Source: CAD feature listing. Evaluate the final solid. Frame: model axes, mm. Face numbers are marked on the shaded views. A direction names the side the tool comes from. Round coordinates to 2 decimals unless told otherwise and drop trailing zeros. Order: outer loops, then holes, each group sorted by start corner. A loop starts at its lowest first (then second) coordinate and runs counter-clockwise, first axis right, second up. Notation, with made-up numbers: M -40,-19 L 8,-19 A37 ccw 8,20 Z; hole C -2.75,52 d2. An arc over 180 degrees is marked long. Answer as CSV lines item,"result". Start each with the question number.
Item 1: Set-up query: the marked faces 1, 2, 3, 4 and 5. Return all of +Z, -Z, +X, -X, +Y, -Y with unobstructed straight access to the full face (end or side cutting, diameter ignored); none if empty.
Item 2: First-contact query: P1, Ø1, axis at x = -54, y = 23, coming from the +Z side; P2, Ø5.5, axis at x = -62.5, z = 3.5, coming from the -Y side; P3, Ø9, axis at x = -55, y = 24, coming from the -Z side; P4, Ø2, axis at y = 43.5, z = 7, coming from the +X side. Flat tips, straight axial feed; report the tip coordinate or a pass-through.
Item 3: Section query B-B on y = 5. Return the cut outline in (x, z), plus the area to 3 significant figures.
Item 4: Section query D-D on y = 24. Return the cut outline in (x, z).
Item 5: Section query C-C on x = -44. Return the cut outline in (y, z).
Item 6: Line query: line 1 (Z direction, x = -56.5, y = 35.5); line 2 (X direction, y = 54.5, z = 1.75); line 3 (Y direction, x = -68, z = 2). Output: solid intervals per line, ascending. Write a range as [from, to].
Item 7: Section query A-A on z = -0.75. Return the cut outline in (x, y), plus the area to 3 significant figures.
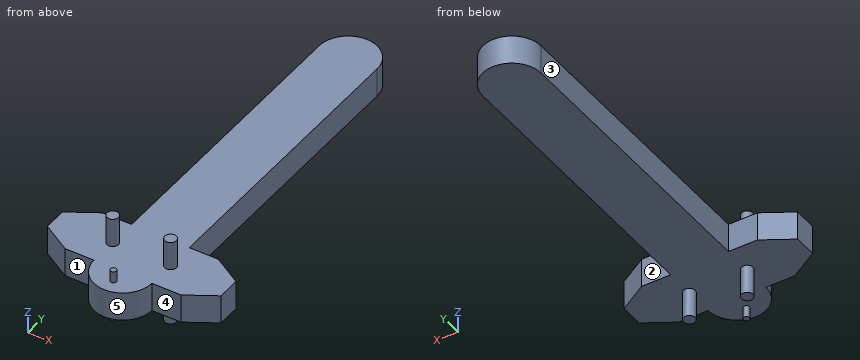
from build123d import *

# Parameters (mm, degrees)
F0_R     = 1
F0_R_2   = 0.5
F1_DEPTH = 5
F2_DEPTH = 7
F3_DEPTH = 2
F4_DEPTH = 10
F5_DEPTH = 5


with BuildPart() as f1:
    # F0 (on Top) → F1 (new body)
    with BuildSketch(Plane.XY):
        with BuildLine():
            Line((-60.480928, 60), (-60.480928, 10))
            Line((-60.480928, 10), (-50.480928, 10))
            Line((-50.480928, 10), (-50.480928, 60))
            ThreePointArc((-50.480928, 60), (-55.480928, 65), (-60.480928, 60))
        make_face()
        Polygon((-50.480928, 10), (-60.480928, 10), (-65.480928, 10), (-70.480928, 7), (-70.480928, 3), (-65.480928, 0), (-60.480928, 0), (-50.480928, 0), (-45.480928, 0), (-40.480928, 3), (-40.480928, 7), (-45.480928, 10), align=None)
        with Locations((-60.480928, 5)):
            Circle(F0_R, mode=Mode.SUBTRACT)
        with Locations((-50.480928, 5)):
            Circle(F0_R, mode=Mode.SUBTRACT)
        with BuildLine():
            Line((-50.480928, 0), (-60.480928, 0))
            ThreePointArc((-60.480928, 0), (-55.480928, -5), (-50.480928, 0))
        make_face()
        with Locations((-55.480928, -2.5)):
            Circle(F0_R_2, mode=Mode.SUBTRACT)
        with Locations((-55.480928, -2.5)):
            Circle(F0_R_2)
    extrude(amount=F1_DEPTH)

    # F0 (on Top) → F2 (join)
    with BuildSketch(Plane.XY):
        with Locations((-55.480928, -2.5)):
            Circle(F0_R_2)
    extrude(amount=F2_DEPTH)

    # F0 (on Top) → F3 (join)
    with BuildSketch(Plane.XY):
        with Locations((-55.480928, -2.5)):
            Circle(F0_R_2)
    extrude(amount=-F3_DEPTH)

    # F0 (on Top) → F4 (join)
    with BuildSketch(Plane.XY):
        with Locations((-60.480928, 5)):
            Circle(F0_R)
        with Locations((-50.480928, 5)):
            Circle(F0_R)
    extrude(amount=F4_DEPTH)

    # F0 (on Top) → F5 (join)
    with BuildSketch(Plane.XY):
        with Locations((-50.480928, 5)):
            Circle(F0_R)
        with Locations((-60.480928, 5)):
            Circle(F0_R)
    extrude(amount=-F5_DEPTH)


solid = f1.part
Results:
1,face 1,"+Z, -Z, -X, -Y"
1,face 2,"+Z, -Z, +X, +Y"
1,face 3,"+Z, -Z, -X, +Y"
1,face 4,"+Z, -Z, +X, -Y"
1,face 5,"+Z, -Z, -Y"
2,P1,"z = 5"
2,P2,"y = -2.6"
2,P3,"z = 0"
2,P4,"through"
3,outline,"M -70.48,0 L -61.48,0 L -61.48,-5 L -59.48,-5 L -59.48,0 L -51.48,0 L -51.48,-5 L -49.48,-5 L -49.48,0 L -40.48,0 L -40.48,5 L -49.48,5 L -49.48,10 L -51.48,10 L -51.48,5 L -59.48,5 L -59.48,10 L -61.48,10 L -61.48,5 L -70.48,5 Z"
3,area,"190 mm^2"
4,outline,"M -60.48,0 L -50.48,0 L -50.48,5 L -60.48,5 Z"
5,outline,"M 0.89,0 L 9.11,0 L 9.11,5 L 0.89,5 Z"
6,line 1,"[0, 5]"
6,line 2,"[-60.48, -50.48]"
6,line 3,"[1.51, 8.49]"
7,outline,"C -60.48,5 d2; C -55.48,-2.5 d1; C -50.48,5 d2"
7,area,"7.07 mm^2"
